Source: CAD feature listing. Evaluate the final solid. Frame: model axes, mm. A direction names the side the tool comes from. Give positions to 0.01 mm unless a question says otherwise; leave off trailing zeros. Order: outer loops, then holes, each group sorted by start corner. A loop starts at its lowest first (then second) coordinate and runs counter-clockwise, first axis right, second up. Notation, with made-up numbers: (-34.75, 14.5) - (-15.75, 14.5) arc R23 cw to (-15.75, 43.5) - close; hole circle Ø5 at (6.5, 3). An arc over 180 degrees is marked (long way). Use CSV: the item, a comma, the result in double quotes.
Autodesk Inventor part; units mm, degrees
ref_plane "YZ Plane" through (0, 0, 0) normal (1, 0, 0) x (0, 1, 0)
ref_plane "XZ Plane" through (0, 0, 0) normal (0, 1, 0) x (-1, 0, 0)
ref_plane "XY Plane" through (0, 0, 0) normal (0, 0, 1) x (1, 0, 0)
sketch "Sketch1" plane through (0, 0, 0) normal (0, 1, 0) x (-1, 0, 0)
  circle A0 centre (0, 0) radius 7.366
  dimension "d0" = 14.732
extrude "Extrusion1" add sketch "Sketch1" along normal blind 6.096
sketch "Sketch2" plane through (0, 6.096, 0) normal (0, 1, 0) x (1, 0, 0)
  circle A0 centre (0, 0) radius 4.191
  dimension "d3" = 8.382
extrude "Extrusion2" add sketch "Sketch2" along normal blind 50.8
sketch "Sketch3" plane through (0, 0, 0) normal (0, -1, 0) x (1, 0, 0)
  circle A0 centre (0, 0) radius 7.366
  circle A1 centre (0, 0) radius 4.191
  circle A2 centre (0, 0) radius 6.096
  circle A3 centre (0, 0) radius 7.366
  dimension "d6" = 12.192
extrude "Extrusion3" cut sketch "Sketch3" against normal through all contours A0
sketch "Sketch4" plane through (0, 56.896, 0) normal (0, 1, 0) x (1, 0, 0)
  circle A0 centre (0, 0) radius 4.191
  circle A1 centre (0, 0) radius 1.905
  dimension "d9" = 3.81
extrude "Extrusion4" cut sketch "Sketch4" against normal through all contours A1
properties part number "arm connector"
Item 1: Section A-A on z = 0. Return the cut outline in (x, y) (3 decimals), then the cut area to 3 significant figures.
Filled in:
outline,"(-6.096, 0) - (-1.905, 0) - (-1.905, 56.896) - (-4.191, 56.896) - (-4.191, 6.096) - (-6.096, 6.096) - close; (1.905, 0) - (6.096, 0) - (6.096, 6.096) - (4.191, 6.096) - (4.191, 56.896) - (1.905, 56.896) - close"
area,"283 mm2"
Item 2: Set-up query: faces 1 (the cylindrical face through (3.997, 31.14, 1.259)), 2 (the flat face through (2, 56.896, 1)). Return all of +Z, -Z, +X, -X, +Y, -Y with unobstructed straight access to the full face (end or side cutting, diameter ignored); none if empty.
Filled in:
face 1,"+Y"
face 2,"+Z, -Z, +X, -X, +Y"
Item 3: Section D-D on x = 5.25. Return the cut outline in (y, z), then the cut area to 3 significant figures.
Filled in:
outline,"(0, -3.1) - (6.1, -3.1) - (6.1, 3.1) - (0, 3.1) - close"
area,"37.8 mm2"
Item 4: Material intervals for line 1 (X direction, y = 25, z = 0) (3 decimals); line 2 (X direction, y = 51, z = -0.5); line 3 (Z direction, x = -1, y = 5), sorted ascending. Write a range as from..to.
Filled in:
line 1,"x = -4.191..-1.905, 1.905..4.191"
line 2,"x = -4.16..-1.84, 1.84..4.16"
line 3,"z = -6.01..-1.62, 1.62..6.01"
Item 5: Mould query, pull axis X, two halves, no side actions, for faces 3 (the flat face through (1.44, 6.096, 4.15)), 4 (the cylindrical face through (-0.41, 28.85, 1.86)), 5 (the cylindrical face through (-0.794, 3.005, 6.044)). Classes: released by +X, released by -X, zero draft, split by the parting line, or undercut.
Filled in:
face 3,"zero draft"
face 4,"undercut"
face 5,"split by the parting line"
Item 6: First-contact query: pin 1 (2 mm diameter, centred on x = 1, y = 30.5, fed in from +Z); pin 2 (3 mm diameter, centred on x = 0.5, y = 23.5, fed in from -Z); pin 3 (4 mm diameter, centred on y = 13.5, z = 3, fed in from -X). Flat tips, straight axial feed; report the tip coordinate or a pass-through.
Filled in:
pin 1,"stops at z = 4.19"
pin 2,"stops at z = -4.19"
pin 3,"stops at x = -4.07"
Item 7: Section B-B on x = 0. Return the cut outline in (y, z) (3 decimals), then the cut area to 3 significant figures.
Filled in:
outline,"(0, -6.096) - (6.096, -6.096) - (6.096, -4.191) - (56.896, -4.191) - (56.896, -1.905) - (0, -1.905) - close; (0, 1.905) - (56.896, 1.905) - (56.896, 4.191) - (6.096, 4.191) - (6.096, 6.096) - (0, 6.096) - close"
area,"283 mm2"
Item 8: Section C-C on y = 11.5. Return the cut outline in (x, z) (3 decimals), then the cut area to 3 significant figures.
Filled in:
outline,"circle Ø8.382 at (0, 0); hole circle Ø3.81 at (0, 0)"
area,"43.8 mm2"
